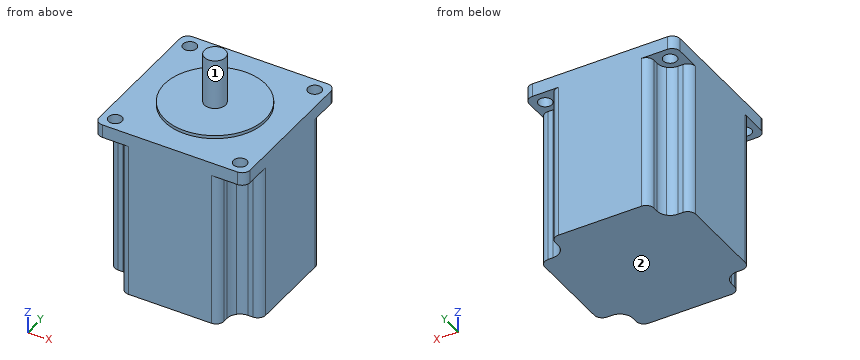
Autodesk Inventor part; units mm, degrees
ref_plane "YZ Plane" through (0, 0, 0) normal (1, 0, 0) x (0, 1, 0)
ref_plane "XZ Plane" through (0, 0, 0) normal (0, 1, 0) x (-1, 0, 0)
ref_plane "XY Plane" through (0, 0, 0) normal (0, 0, 1) x (1, 0, 0)
sketch "Sketch1" plane through (0, 0, 0) normal (0, 0, 1) x (1, 0, 0)
  line L0 (-28.5, -28.5) -> (28.5, -28.5)
  line L1 (28.5, -28.5) -> (28.5, 28.5)
  line L2 (28.5, 28.5) -> (-28.5, 28.5)
  line L3 (-28.5, 28.5) -> (-28.5, -28.5)
  line L4 (-28.5, -28.5) -> (28.5, 28.5) construction
  line L5 (28.5, -28.5) -> (-28.5, 28.5) construction
  circle A0 centre (23.57, 23.57) radius 2.55
  line L6 (0, 28.5) -> (0, -28.5) construction
  line L7 (28.5, 0) -> (-28.5, 0) construction
  circle A1 centre (-23.57, 23.57) radius 2.55
  circle A2 centre (23.57, -23.57) radius 2.55
  circle A3 centre (-23.57, -23.57) radius 2.55
  circle A4 centre (0, 0) radius 19.05
  circle A5 centre (0, 0) radius 4
  dimension "d0" = 57
  dimension "d1" = 57
  dimension "d2" = 5.1
  dimension "d3" = 47.14
  dimension "d4" = 38.1
  dimension "d5" = 8
extrude "Extrusion1" add sketch "Sketch1" against normal blind 64 contours L3 L2 L1 L0 | A4 | A5
extrude "Extrusion2" add sketch "Sketch1" along normal blind 1.2 contours A4
extrude "Extrusion3" add sketch "Sketch1" along normal blind 20.2 contours A5
sketch "Sketch2" plane through (0, 0, -64) normal (0, 0, -1) x (-1, 0, 0)
  circle A0 centre (-23.57, -23.57) radius 2.55
  circle A1 centre (23.57, -23.57) radius 2.55
  circle A2 centre (23.57, 23.57) radius 2.55
  circle A3 centre (-23.57, 23.57) radius 2.55
  line L0 (-28.5, -28.5) -> (28.5, -28.5)
  line L1 (28.5, -28.5) -> (28.5, 28.5)
  line L2 (28.5, 28.5) -> (-28.5, 28.5)
  line L3 (-28.5, 28.5) -> (-28.5, -28.5)
  line L4 (-28.5, -28.5) -> (-28.5, 28.5)
  line L5 (28.5, 28.5) -> (28.5, -28.5)
  line L6 (-18.64, -18.64) -> (-23.57, -18.64) construction
  line L7 (-28.5, -18.64) -> (-28.5, -28.5)
  line L8 (-28.5, -28.5) -> (-18.64, -28.5)
  line L9 (-18.64, -28.5) -> (-18.64, -23.57)
  line L10 (-18.64, -18.64) -> (-28.5, -28.5) construction
  line L11 (-28.5, -18.64) -> (-18.64, -28.5) construction
  line L12 (-28.5, 28.5) -> (28.5, 28.5)
  circle A4 centre (-23.57, -23.57) radius 2.55
  arc A5 (-27.056, -20.084) -> (-28.5, -23.57) centre (-23.57, -23.57) ccw construction
  line L13 (-18.64, -23.57) -> (-18.64, -18.64) construction
  line L14 (-23.57, -18.64) -> (-28.5, -18.64)
  arc A6 (-23.57, -18.64) -> (-27.056, -20.084) centre (-23.57, -23.57) ccw construction
  arc A7 (-27.056, -27.056) -> (-20.084, -27.056) centre (-23.57, -23.57) ccw construction
  arc A8 (-20.084, -27.056) -> (-18.64, -23.57) centre (-23.57, -23.57) ccw construction
  arc A9 (-20.084, -20.084) -> (-23.57, -18.64) centre (-23.57, -23.57) ccw
  arc A10 (-18.64, -23.57) -> (-20.084, -20.084) centre (-23.57, -23.57) ccw
  arc A11 (-28.5, -23.57) -> (-27.056, -27.056) centre (-23.57, -23.57) ccw construction
  line L15 (0, 28.5) -> (0, -28.5) construction
  line L16 (-28.5, -28.5) -> (28.5, -28.5) construction
  line L17 (28.5, 0) -> (-28.5, 0) construction
  circle A12 centre (23.57, -23.57) radius 2.55
  line L18 (18.64, -18.64) -> (23.57, -18.64) construction
  line L19 (28.5, -18.64) -> (28.5, -28.5)
  line L20 (28.5, -28.5) -> (18.64, -28.5)
  line L21 (18.64, -28.5) -> (18.64, -23.57)
  line L22 (18.64, -18.64) -> (28.5, -28.5) construction
  line L23 (28.5, -18.64) -> (18.64, -28.5) construction
  circle A13 centre (23.57, -23.57) radius 2.55
  arc A14 (28.5, -23.57) -> (27.056, -20.084) centre (23.57, -23.57) ccw construction
  line L24 (18.64, -23.57) -> (18.64, -18.64) construction
  line L25 (23.57, -18.64) -> (28.5, -18.64)
  arc A15 (27.056, -20.084) -> (23.57, -18.64) centre (23.57, -23.57) ccw construction
  arc A16 (20.084, -27.056) -> (27.056, -27.056) centre (23.57, -23.57) ccw construction
  arc A17 (18.64, -23.57) -> (20.084, -27.056) centre (23.57, -23.57) ccw construction
  arc A18 (23.57, -18.64) -> (20.084, -20.084) centre (23.57, -23.57) ccw
  arc A19 (20.084, -20.084) -> (18.64, -23.57) centre (23.57, -23.57) ccw
  arc A20 (27.056, -27.056) -> (28.5, -23.57) centre (23.57, -23.57) ccw construction
  circle A21 centre (-23.57, 23.57) radius 2.55
  circle A22 centre (23.57, 23.57) radius 2.55
  line L26 (-18.64, 18.64) -> (-23.57, 18.64) construction
  line L27 (-28.5, 18.64) -> (-28.5, 28.5)
  line L28 (-28.5, 28.5) -> (-18.64, 28.5)
  line L29 (-18.64, 28.5) -> (-18.64, 23.57)
  line L30 (-18.64, 18.64) -> (-28.5, 28.5) construction
  line L31 (-28.5, 18.64) -> (-18.64, 28.5) construction
  circle A23 centre (-23.57, 23.57) radius 2.55
  arc A24 (-28.5, 23.57) -> (-27.056, 20.084) centre (-23.57, 23.57) ccw construction
  line L32 (-18.64, 23.57) -> (-18.64, 18.64) construction
  line L33 (-23.57, 18.64) -> (-28.5, 18.64)
  arc A25 (-27.056, 20.084) -> (-23.57, 18.64) centre (-23.57, 23.57) ccw construction
  arc A26 (-20.084, 27.056) -> (-27.056, 27.056) centre (-23.57, 23.57) ccw construction
  arc A27 (-18.64, 23.57) -> (-20.084, 27.056) centre (-23.57, 23.57) ccw construction
  arc A28 (-23.57, 18.64) -> (-20.084, 20.084) centre (-23.57, 23.57) ccw
  arc A29 (-20.084, 20.084) -> (-18.64, 23.57) centre (-23.57, 23.57) ccw
  arc A30 (-27.056, 27.056) -> (-28.5, 23.57) centre (-23.57, 23.57) ccw construction
  line L34 (-28.5, 28.5) -> (28.5, 28.5) construction
  circle A31 centre (23.57, 23.57) radius 2.55
  line L35 (18.64, 23.57) -> (18.64, 18.64) construction
  arc A32 (18.64, 23.57) -> (20.084, 20.084) centre (23.57, 23.57) ccw
  line L36 (18.64, 28.5) -> (18.64, 23.57)
  line L37 (18.64, 18.64) -> (23.57, 18.64) construction
  arc A33 (20.084, 27.056) -> (18.64, 23.57) centre (23.57, 23.57) ccw construction
  arc A34 (20.084, 20.084) -> (23.57, 18.64) centre (23.57, 23.57) ccw
  arc A35 (23.57, 18.64) -> (27.056, 20.084) centre (23.57, 23.57) ccw construction
  line L38 (23.57, 18.64) -> (28.5, 18.64)
  arc A36 (27.056, 20.084) -> (28.5, 23.57) centre (23.57, 23.57) ccw construction
  arc A37 (27.056, 27.056) -> (20.084, 27.056) centre (23.57, 23.57) ccw construction
  arc A38 (28.5, 23.57) -> (27.056, 27.056) centre (23.57, 23.57) ccw construction
  line L39 (28.5, 18.64) -> (28.5, 28.5)
  line L40 (18.64, 18.64) -> (28.5, 28.5) construction
  line L41 (28.5, 18.64) -> (18.64, 28.5) construction
  line L42 (28.5, 28.5) -> (18.64, 28.5)
  circle A39 centre (23.57, 23.57) radius 2.55
  point P0 (0, 0)
extrude "Extrusion4" cut sketch "Sketch2" against normal blind 59 contours L3 L14 A9 A10 L9 L0 | L21 A19 A18 L25 L1 L0 | L3 L2 L29 A29 A28 L33 | L38 A34 A32 L36 L2 L1
fillet "Fillet1" radius 3 12 edges at (28.5, 28.5, -2.5) (-28.5, 28.5, -2.5) (-28.5, -28.5, -2.5) (28.5, -28.5, -2.5) (-18.64, -28.5, -34.5) (-28.5, -18.64, -34.5) (18.64, -28.5, -34.5) (28.5, -18.64, -34.5) (28.5, 18.64, -34.5) (18.64, 28.5, -34.5) (-18.64, 28.5, -34.5) (-28.5, 18.64, -34.5)
properties part number "nema23-wotiom"
Can you work these out from the model? Positions are in its coordinate system, mm. Face numbers are marked on the shaded views. A direction names the side the tool comes from. Coordinates: 2 decimals unless noted, no trailing zeros. Order: outer loops, then holes, each group sorted by start corner. A loop starts at its lowest first (then second) coordinate and runs counter-clockwise, first axis right, second up. Notation, with made-up numbers: (-33.5, -14) - (-5.5, -14) arc R27 ccw to (-5.5, 18) - close; hole circle Ø3 at (80, 17.25). An arc over 180 degrees is marked (long way). Answer as a JSON object with one key per item and string values. Group by question number.
Q1. Imagine slicing it at A-A (y = 0). Please give me the cut outline in (x, z).
Q2. On a 3-axis mill with a long thin cutter (end or side, diameter ignored), from which of +Z, -Z, +X, -X, +Y, -Y can I reach the whole of each face in a straight line? I mean the marked faces 1 and 2. Say none if no direction works.
Q3. I need wall thicknesses on line 1 (X direction, y = 23.57, z = -3.95); line 2 (X direction, y = 23, z = -1). Which ranges of each line are inside material? Lowest first, please. Write a range as from..to.
Q4. Imagine slicing it at C-C (z = -3). Please give me the cut outline in (x, y), and give its area (3 significant figures).
Q5. Will these pins go through, and if not, where does the flat tip stop? P1, Ø1.5, axis at x = -24, z = -46.5, coming from the -Y side; P2, Ø1.5, axis at y = -24.5, z = -35, coming from the +X side; P3, Ø1, axis at x = 17.5, z = -26, coming from the -Y side; P4, Ø3, axis at y = 16.5, z = -6, coming from the -X side.
Q6. Imagine slicing it at B-B (z = -31.5). Please give me the cut outline in (x, y).
Determined:
{
 "1": {"outline": "(-28.5, -64) - (28.5, -64) - (28.5, 0) - (19.05, 0) - (19.05, 1.2) - (4, 1.2) - (4, 20.2) - (-4, 20.2) - (-4, 1.2) - (-19.05, 1.2) - (-19.05, 0) - (-28.5, 0) - close"},
 "2": {"face 1": "+Z", "face 2": "-Z, +X, -X, +Y, -Y"},
 "3": {"line 1": "x = -28.5..-26.12, -21.02..21.02, 26.12..28.5", "line 2": "x = -28.5..-26.06, -21.08..21.08, 26.06..28.5"},
 "4": {"outline": "(-28.5, -25.5) arc R3 ccw to (-25.5, -28.5) - (25.5, -28.5) arc R3 ccw to (28.5, -25.5) - (28.5, 25.5) arc R3 ccw to (25.5, 28.5) - (-25.5, 28.5) arc R3 ccw to (-28.5, 25.5) - close; hole circle Ø5.1 at (-23.57, -23.57); hole circle Ø5.1 at (-23.57, 23.57); hole circle Ø5.1 at (23.57, -23.57); hole circle Ø5.1 at (23.57, 23.57)", "area": "3,160 mm2"},
 "5": {"P1": "stops at y = -18.65", "P2": "stops at x = 18.64", "P3": "stops at y = -28.17", "P4": "stops at x = -28.5"},
 "6": {"outline": "(-28.5, -15.64) arc R3 ccw to (-25.5, -18.64) - (-23.57, -18.64) arc R4.93 cw to (-20.08, -20.08) arc R4.93 cw to (-18.64, -23.57) - (-18.64, -25.5) arc R3 ccw to (-15.64, -28.5) - (15.64, -28.5) arc R3 ccw to (18.64, -25.5) - (18.64, -23.57) arc R4.93 cw to (20.08, -20.08) arc R4.93 cw to (23.57, -18.64) - (25.5, -18.64) arc R3 ccw to (28.5, -15.64) - (28.5, 15.64) arc R3 ccw to (25.5, 18.64) - (23.57, 18.64) arc R4.93 cw to (20.08, 20.08) arc R4.93 cw to (18.64, 23.57) - (18.64, 25.5) arc R3 ccw to (15.64, 28.5) - (-15.64, 28.5) arc R3 ccw to (-18.64, 25.5) - (-18.64, 23.57) arc R4.93 cw to (-20.08, 20.08) arc R4.93 cw to (-23.57, 18.64) - (-25.5, 18.64) arc R3 ccw to (-28.5, 15.64) - close"}
}
